Geometry: final body of the model. Coordinates: model frame, mm. Face numbers are marked on the shaded views. Give positions to 0.01 mm unless a question says otherwise; leave off trailing zeros. Write each loop counter-clockwise with the first axis right and the second up, starting at its lowest first coordinate (ties: lowest second). Pieces come first, ordered by that corner, then holes. Notation, with made-up numbers: (12, -5.5) -> (35, -5.5) arc R26 cw to (35, 19.5) -> close; hole circle Ø1 at (28.25, -1). An arc over 180 degrees is marked (long way). Answer as a JSON object with one key per item and string values. Group by question number.
(1) Material intervals for probe 1 along Z at (x, y) = (19, 2.75); probe 2 along Z at (x, y) = (26.5, 4.5); probe 3 along X at (y, z) = (12.75, -95.5), sorted ascending.
(2) Contact query for flat-ended pins moving along their axis: pin 1 Ø4 at (y, z) = (3.5, -60.5) entering from +X; pin 2 Ø3 at (y, z) = (11, -112.5) entering from -X. Output: stop coordinate, or through.
(3) Section query A-A on x = 6. Output: boundary loops of the cut face in (y, z), plus the area to 3 significant figures.
(4) Draft query along X for the marked faces 1, 2 and 3. Return one class per face: +X half, -X half, draft (parallel to the pull), parting line (faces both ways), or undercut.
(5) Section query C-C on z = 29. Output: boundary loops of the cut face in (x, y), plus the area to 3 significant figures.
(6) Section query D-D on y = 12.25. Output: boundary loops of the cut face in (x, z), plus the area to 3 significant figures.
(7) Section query B-B on z = -98.5. Output: boundary loops of the cut face in (x, y), plus the area to 3 significant figures.
Solid Edge part; units mm, degrees
sketch "Sketch1" plane through (0, 0, 0) normal (0, -1, 0) x (1, 0, 0)
  line L0 (-41.3956, 47.354) -> (78.6044, 47.354)
  line L1 (78.6044, 47.354) -> (78.6044, -2.646)
  line L2 (78.6044, -2.646) -> (43.6044, -132.646)
  line L3 (43.6044, -132.646) -> (-6.3956, -132.646)
  line L4 (-41.3956, -2.646) -> (-6.3956, -132.646)
  line L5 (-41.3956, 47.354) -> (-41.3956, -2.646)
extrude "Protrusion1" add sketch "Sketch1" against normal blind 15
hole "Hole1" at (18.6044, 0, -102.646) direction (0, 1, 0) diameter 30 end up to next
hole "Hole_2" at (48.6044, 0, 22.354) direction (0, 1, 0) diameter 20 end up to next
hole "Hole_3" at (-11.3956, 0, 22.354) direction (0, 1, 0) diameter 20 end up to next
properties part number "SP-2070" material "Steel"
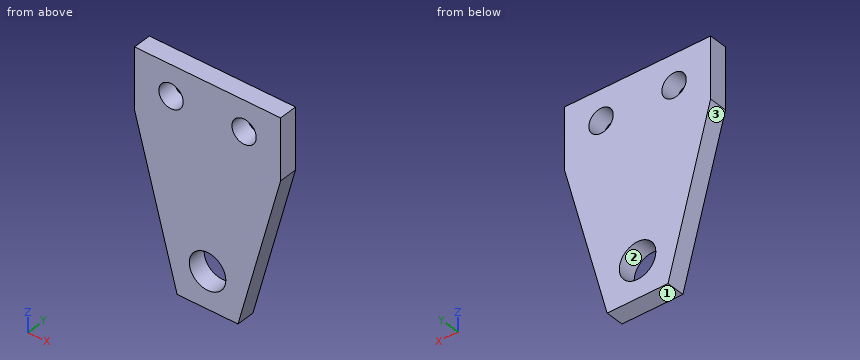
Answer list:
{
 "1": {"probe 1": "-132.65 to -117.64, -87.65 to 47.35", "probe 2": "-132.65 to -115.4, -89.89 to 47.35", "probe 3": "-16.4 to 5.42, 31.79 to 53.61"},
 "2": {"pin 1": "x = 63.57", "pin 2": "x = -12.22"},
 "3": {"outline": "(0, -132.65) -> (15, -132.65) -> (15, -110.78) -> (0, -110.78) -> close; (0, -94.51) -> (15, -94.51) -> (15, 47.35) -> (0, 47.35) -> close", "area": "2,460 mm2"},
 "4": {"face 1": "draft", "face 2": "undercut", "face 3": "-X half"},
 "5": {"outline": "(-41.4, 0) -> (-18.87, 0) -> (-18.87, 15) -> (-41.4, 15) -> close; (-3.92, 0) -> (41.13, 0) -> (41.13, 15) -> (-3.92, 15) -> close; (56.08, 0) -> (78.6, 0) -> (78.6, 15) -> (56.08, 15) -> close", "area": "1,350 mm2"},
 "6": {"outline": "(-41.4, -2.65) -> (-6.4, -132.65) -> (43.6, -132.65) -> (78.6, -2.65) -> (78.6, 47.35) -> (-41.4, 47.35) -> close; hole circle Ø20 at (-11.4, 22.35); hole circle Ø30 at (18.6, -102.65); hole circle Ø20 at (48.6, 22.35)", "area": "15,700 mm2"},
 "7": {"outline": "(-15.59, 0) -> (4.19, 0) -> (4.19, 15) -> (-15.59, 15) -> close; (33.02, 0) -> (52.8, 0) -> (52.8, 15) -> (33.02, 15) -> close", "area": "593 mm2"}
}
